Autodesk Inventor part; units mm, degrees
ref_plane "YZ Plane" through (0, 0, 0) normal (1, 0, 0) x (0, 1, 0)
ref_plane "XZ Plane" through (0, 0, 0) normal (0, 1, 0) x (-1, 0, 0)
ref_plane "XY Plane" through (0, 0, 0) normal (0, 0, 1) x (1, 0, 0)
sketch "Sketch1" plane through (0, 0, 0) normal (0, 0, 1) x (1, 0, 0)
  line L0 (0, 0) -> (0, 9.5)
  line L1 (0, 9.5) -> (12, 9.5)
  line L2 (12, 9.5) -> (12, 0)
  line L3 (12, 0) -> (7.25, 0)
  line L4 (7.25, 0) -> (7.25, 6.5)
  line L5 (7.25, 6.5) -> (4.75, 6.5)
  line L6 (4.75, 6.5) -> (4.75, 0)
  line L7 (4.75, 0) -> (0, 0)
  line L8 (6, 6.5) -> (6, 0.5) construction
  dimension "d17" = 6.5
  dimension "d18" = 12
  dimension "d20" = 2.5
  dimension "d21" = 3
extrude "Extrusion1" add sketch "Sketch1" along normal blind 7
sketch "Sketch3" plane through (7.25, 0, 0) normal (0, -1, 0) x (1, 0, 0)
  line L0 (-2.5, 0) -> (0, 0)
  line L1 (0, 0) -> (0, 7)
  line L2 (-2.5, 7) -> (0, 7)
  line L3 (-2.5, 0) -> (-2.5, 7)
  line L4 (0, 0) -> (4.75, 0)
  line L5 (4.75, 0) -> (4.75, 7)
  line L6 (0, 7) -> (4.75, 7)
  line L7 (0, 0) -> (0, 7)
  line L8 (-7.25, 0) -> (-2.5, 0)
  line L9 (-2.5, 0) -> (-2.5, 7)
  line L10 (-7.25, 7) -> (-2.5, 7)
  line L11 (-7.25, 0) -> (-7.25, 7)
  line L12 (-7.25, 21.16) -> (4.75, 21.16)
  line L13 (4.75, 21.16) -> (4.75, 8.38)
  line L14 (4.75, 8.38) -> (-7.25, 8.38)
  line L15 (-7.25, 8.38) -> (-7.25, 21.16)
  line L16 (4.75, 8.38) -> (4.25, 7.63)
  line L17 (4.25, 7.63) -> (3.75, 8.38)
  line L18 (4.75, 0) -> (4.75, 7)
  line L19 (-7.25, 0) -> (-7.25, 7)
  line L20 (-1.25, 8.38) -> (-1.25, 21.16) construction
  line L21 (2.75, 8.38) -> (2.25, 7.63)
  line L22 (2.25, 7.63) -> (1.75, 8.38)
  line L23 (0.75, 8.38) -> (0.25, 7.63)
  line L24 (0.25, 7.63) -> (-0.25, 8.38)
  line L25 (-1.25, 8.38) -> (-1.75, 7.63)
  line L26 (-1.75, 7.63) -> (-2.25, 8.38)
  line L27 (-3.25, 8.38) -> (-3.75, 7.63)
  line L28 (-3.75, 7.63) -> (-4.25, 8.38)
  line L29 (-5.25, 8.38) -> (-5.75, 7.63)
  line L30 (-5.75, 7.63) -> (-6.25, 8.38)
  circle A0 centre (-1.25, 15.16) radius 6
  line L31 (-5.4926, 19.4026) -> (-7.25, 17.6453)
  line L32 (2.9926, 19.4026) -> (4.75, 17.6453)
  point P0 (-6.25, 8.38)
  point P1 (-5.25, 8.38)
  point P2 (-4.25, 8.38)
  point P3 (-3.25, 8.38)
  point P4 (-2.25, 8.38)
  point P5 (-1.25, 8.38)
  point P6 (-0.25, 8.38)
  point P7 (0.75, 8.38)
  point P8 (1.75, 8.38)
  dimension "d22" = 1.38
  dimension "d23" = 12.78
  dimension "d24" = 0.75
  dimension "d25" = 1
  dimension "d28" = 2
  dimension "d42" = 12
  dimension "d43" = 135
  dimension "d44" = 135
extrude "Extrusion2" add sketch "Sketch3" against normal up to surface (9.5 mm away) contours A0 | L31 A0 L15 | L32 L13 A0 | A0 L13 L14 L15 | L16 L17 L14 | L14 L29 L30 | L21 L22 L14 | L14 L27 L28 | L23 L24 L14 | L14 L25 L26
fillet "Fillet2" radius 1 2 edges at (4.75, 3.25, 7) (7.25, 3.25, 7)
fillet "Fillet3" radius 2 4 edges at (12, 4.75, 0) (0, 4.75, 0) (7.25, 3.25, 0) (4.75, 3.25, 0)
chamfer "Chamfer1" distance 0.3 angle 45 6 edges at (11.5, 4.75, 7.63) (9.5, 4.75, 7.63) (7.5, 4.75, 7.63) (5.5, 4.75, 7.63) (3.5, 4.75, 7.63) (1.5, 4.75, 7.63)
sketch "Sketch5" plane through (6, 9.5, 15.16) normal (0, 1, 0) x (1, 0, 0)
  line L0 (-4.6664, 7.2804) -> (-4.3336, 7.2804)
  line L1 (-5, 6.78) -> (-4.6664, 7.2804)
  line L2 (-6, 6.78) -> (-5, 6.78)
  line L3 (-6, -2.4853) -> (-6, 6.78)
  line L4 (-4.2426, -4.2426) -> (-6, -2.4853)
  arc A0 (-4.2426, -4.2426) -> (4.2426, -4.2426) centre (0, 0) ccw
  line L5 (6, -2.4853) -> (4.2426, -4.2426)
  line L6 (6, 6.78) -> (6, -2.4853)
  line L7 (5.6664, 7.2804) -> (6, 6.78)
  line L8 (5.3336, 7.2804) -> (5.6664, 7.2804)
  line L9 (5, 6.78) -> (5.3336, 7.2804)
  line L10 (4, 6.78) -> (5, 6.78)
  line L11 (3.6664, 7.2804) -> (4, 6.78)
  line L12 (3.3336, 7.2804) -> (3.6664, 7.2804)
  line L13 (3, 6.78) -> (3.3336, 7.2804)
  line L14 (2, 6.78) -> (3, 6.78)
  line L15 (1.6664, 7.2804) -> (2, 6.78)
  line L16 (1.3336, 7.2804) -> (1.6664, 7.2804)
  line L17 (1, 6.78) -> (1.3336, 7.2804)
  line L18 (0, 6.78) -> (1, 6.78)
  line L19 (-0.3336, 7.2804) -> (0, 6.78)
  line L20 (-0.6664, 7.2804) -> (-0.3336, 7.2804)
  line L21 (-1, 6.78) -> (-0.6664, 7.2804)
  line L22 (-2, 6.78) -> (-1, 6.78)
  line L23 (-2.3336, 7.2804) -> (-2, 6.78)
  line L24 (-2.6664, 7.2804) -> (-2.3336, 7.2804)
  line L25 (-3, 6.78) -> (-2.6664, 7.2804)
  line L26 (-4, 6.78) -> (-3, 6.78)
  line L27 (-4.3336, 7.2804) -> (-4, 6.78)
  arc A1 (-4, 15.16) -> (-6, 13.16) centre (-4, 13.16) ccw
  line L28 (-6, 13.16) -> (-6, 8.16)
  line L29 (6, 8.16) -> (-6, 8.16)
  line L30 (6, 13.16) -> (6, 8.16)
  arc A2 (6, 13.16) -> (4, 15.16) centre (4, 13.16) ccw
  line L31 (4, 15.16) -> (-4, 15.16)
  line L32 (-6, -2.4853) -> (-6, 6.78)
  line L33 (-6, 6.78) -> (-6, 11.1694)
  line L34 (6, 6.78) -> (6, 8.16)
  point P0 (-6, 15.16)
extrude "Extrusion4" add sketch "Sketch5" against normal up to surface (3 mm away)
sketch "Sketch7" plane through (6, 9.5, 15.16) normal (0, 1, 0) x (1, 0, 0)
  circle A0 centre (0, 0) radius 3
  arc A1 (-4.2426, -4.2426) -> (4.2426, -4.2426) centre (0, 0) ccw
  point P0 (-6, 15.16)
  dimension "d48" = 6
extrude "Extrusion5" cut sketch "Sketch7" against normal blind 5.5
sketch "Sketch8" plane through (6, 4, 15.16) normal (0, 1, 0) x (1, 0, 0)
  circle A0 centre (0, 0) radius 3
  point P0 (-6, 15.16)
hole "Hole2" at (6, 4, 15.16) direction (0, -1, 0) diameter 3.4 end through all
chamfer "Chamfer2" distance 1.3 angle 45 1 edges at (6, 4, 13.46)
properties part number "Belt Clip"
The listing builds one solid part. Answer for the finished solid, in the listing's coordinates (mm). A direction names the side the tool comes from. Coordinates: 2 decimals unless noted, no trailing zeros. Loops run counter-clockwise (first coordinate to the right, second up) from the corner with the lowest first, then second, coordinate; pieces in that order, holes last. Notation, with made-up numbers: M 68.25,28 L 121.25,28 A29 cw 121.25,65 Z; hole C -11,27 d3. An arc over 180 degrees is marked long. Answer as a JSON object with one key per item and string values. Group by question number.
Item 1: Section D-D (x = 2.25) is taken. Write down the section's boundary in (y, z), and give its area (3 significant figures).
Item 2: Section B-B (y = 8.25) is taken. Write down the section's boundary in (x, z), and give its area (3 significant figures).
Item 3: Determine the mould class of faces 1 (the face through (10.5, 3.2, 8.38)), 2 (the face through (11.4, 4.68, 0.57)), 3 (the face through (2, 0, 3)), 4 (the face through (0.891, 4.684, 18.536)) for opening direction X: +X half, -X half, draft (parallel to the pull), parting line (faces both ways), or undercut.
Item 4: Which of the six approach directions +Z, -Z, +X, -X, +Y, -Y give full straight-line access (tool end or side, diameter ignored) to faces 5 (the face through (8.77, 6.79, 16.31)), 6 (the face through (10, 3, 7)), 7 (the face through (8.5, 3.2, 8.38)), 8 (the face through (6.5, 3.2, 8.38))?
Item 5: Consider L1, parallel to X at y = 4.75, z = 3.75; L2, parallel to X at y = 6.85, z = 15.16; L3, parallel to Z at x = 6, y = 6.7. Determine where each line is inside the solid, lowest interval first.
Item 6: Each of these flat-tipped pins is pushed along its axis until it touches: P1, Ø3, axis at x = 5.5, z = 16, coming from the +Y side; P2, Ø2.5, axis at x = 6, z = 15.16, coming from the +Y side; P3, Ø4, axis at x = 11, y = 2, coming from the +Z side; P4, Ø0.5, axis at x = 4.5, y = 2, coming from the -Z side. Where does it stop, or does it pass through?
Item 7: Section C-C (z = 2.75) is taken. Write down the section's boundary in (x, y), and give its area (4 significant figures).
Solved:
{
 "1": {"outline": "M 0,0 L 9.5,0 L 9.5,19.84 L 0,19.84 L 0,8.38 L 6.5,8.38 L 6.5,7 L 0,7 Z", "area": "180 mm2"},
 "2": {"outline": "M 0,2 A2 ccw 2,0 L 10,0 A2 ccw 12,2 L 12,17.65 L 10.24,19.4 A6 ccw 1.76,19.4 L 0,17.65 Z; hole C 6,15.16 d6", "area": "210 mm2"},
 "3": {"face 1": "undercut", "face 2": "+X half", "face 3": "draft", "face 4": "-X half"},
 "4": {"face 5": "+Y", "face 6": "+X, -X, -Y", "face 7": "-Y", "face 8": "-Z, -Y"},
 "5": {"L1": "x = 0 to 4.75, 7.25 to 12", "L2": "x = 0 to 3, 9 to 12", "L3": "z = 0 to 12.16, 18.16 to 21.16"},
 "6": {"P1": "stops at y = 3.48", "P2": "passes through", "P3": "stops at z = 20.36", "P4": "stops at z = 0.68"},
 "7": {"outline": "M 0,0 L 4.75,0 L 4.75,6.5 L 7.25,6.5 L 7.25,0 L 12,0 L 12,9.5 L 0,9.5 Z", "area": "97.75 mm2"}
}
